The listing builds one solid part. Answer for the finished solid, in the listing's coordinates (mm). A direction names the side the tool comes from. Give positions to 0.01 mm unless a question says otherwise; leave off trailing zeros. Order: outer loops, then holes, each group sorted by start corner. A loop starts at its lowest first (then second) coordinate and runs counter-clockwise, first axis right, second up. Notation, with made-up numbers: (-16.75, -14.5) - (22.25, -14.5) arc R10 ccw to (22.25, 1.5) - close; hole circle Ø9 at (-2, 26.25). An arc over 180 degrees is marked (long way). Answer in a Markdown table with one row per item. Add a question column.
Autodesk Inventor part; units mm, degrees
ref_plane "YZ Plane" through (0, 0, 0) normal (1, 0, 0) x (0, 1, 0)
ref_plane "XZ Plane" through (0, 0, 0) normal (0, 1, 0) x (-1, 0, 0)
ref_plane "XY Plane" through (0, 0, 0) normal (0, 0, 1) x (1, 0, 0)
sketch "Sketch1" plane through (0, 0, 0) normal (0, 0, 1) x (1, 0, 0)
  line L0 (80, 30) -> (-80, 30)
  line L1 (-80, 30) -> (-80, -30)
  line L2 (-80, -30) -> (80, -30)
  line L3 (80, -30) -> (80, 30)
  line L4 (80, 30) -> (-80, -30) construction
  line L5 (-80, 30) -> (80, -30) construction
  line L6 (-20, -30) -> (-80, -30)
  line L7 (-80, -30) -> (-80, 30)
  line L8 (-80, 30) -> (-20, 30)
  line L9 (-20, 30) -> (-20, -30)
  line L10 (-20, -30) -> (-80, 30) construction
  line L11 (-80, -30) -> (-20, 30) construction
  line L12 (20, -30) -> (80, -30)
  line L13 (80, -30) -> (80, 30)
  line L14 (80, 30) -> (20, 30)
  line L15 (20, 30) -> (20, -30)
  line L16 (20, -30) -> (80, 30) construction
  line L17 (80, -30) -> (20, 30) construction
  line L18 (0, 30) -> (0, -30) construction
  point P0 (0, 0)
  point P1 (-50, 0)
  point P2 (50, 0)
  point P3 (20, 30)
  point P4 (20, -30)
  point P5 (-20, -30)
  point P6 (-20, 30)
  dimension "d0" = 160
  dimension "d1" = 60
  dimension "d2" = 40
extrude "Extrusion1" add sketch "Sketch1" along normal blind 10 contours L3 L2 L15 L0 | L9 L2 L1 L0
sketch "Sketch2" plane through (0, 0, 10) normal (0, 0, 1) x (1, 0, 0)
  line L0 (-80, -30) -> (-20, -30)
  line L1 (80, -24) -> (-80, -24)
  line L2 (-80, -24) -> (-80, -30)
  line L3 (-80, -30) -> (80, -30)
  line L4 (80, -30) -> (80, -24)
  line L5 (80, -24) -> (-80, -30) construction
  line L6 (-80, -24) -> (80, -30) construction
  line L7 (80, -30) -> (80, 30)
  point P0 (0, 0)
  point P1 (0, -27)
  dimension "d5" = 6
extrude "Extrusion2" add sketch "Sketch2" along normal blind 115
sketch "Sketch3" plane through (0, 0, 0) normal (0, 0, -1) x (-1, 0, 0)
  line L0 (53, 7.5) -> (43, 7.5)
  line L1 (43, 7.5) -> (43, -7.5)
  line L2 (43, -7.5) -> (53, -7.5)
  line L3 (53, -7.5) -> (53, 7.5)
  line L4 (53, 7.5) -> (43, -7.5) construction
  line L5 (43, 7.5) -> (53, -7.5) construction
  line L6 (-43, 7.5) -> (-53, 7.5)
  line L7 (-53, 7.5) -> (-53, -7.5)
  line L8 (-53, -7.5) -> (-43, -7.5)
  line L9 (-43, -7.5) -> (-43, 7.5)
  line L10 (-43, 7.5) -> (-53, -7.5) construction
  line L11 (-53, 7.5) -> (-43, -7.5) construction
  line L12 (80, -30) -> (-80, -30) construction
  line L13 (0, -30) -> (0, 0) construction
  point P0 (48, 0)
  point P1 (-48, 0)
  point P2 (48, 0)
  dimension "d8" = 10
  dimension "d9" = 15
  dimension "d10" = 48
extrude "Extrusion3" cut sketch "Sketch3" against normal through all
sketch "Sketch4" plane through (0, 0, 0) normal (0, 0, -1) x (-1, 0, 0)
  line L0 (-70, -20) -> (70, -20) construction
  line L1 (70, -20) -> (70, 20) construction
  line L2 (70, 20) -> (-70, 20) construction
  line L3 (-70, 20) -> (-70, -20) construction
  line L4 (-70, -20) -> (70, 20) construction
  line L5 (70, -20) -> (-70, 20) construction
  circle A0 centre (70, 20) radius 1.25
  circle A1 centre (-70, 20) radius 1.25
  circle A2 centre (-70, -20) radius 1.25
  circle A3 centre (70, -20) radius 1.25
  point P0 (0, 0)
  dimension "d13" = 140
  dimension "d14" = 40
  dimension "d16" = 2.5
extrude "Extrusion4" cut sketch "Sketch4" against normal through all
sketch "Sketch5" plane through (-20, -24, 10) normal (0, 1, 0) x (1, 0, 0)
  line L0 (59.5, -13) -> (-19.5, -13) construction
  line L1 (-19.5, -13) -> (-19.5, -113) construction
  line L2 (-19.5, -113) -> (59.5, -113) construction
  line L3 (59.5, -113) -> (59.5, -13) construction
  line L4 (59.5, -13) -> (-19.5, -113) construction
  line L5 (-19.5, -13) -> (59.5, -113) construction
  line L6 (100, -115) -> (-60, -115) construction
  line L7 (55.5, -17) -> (-2.5, -17) construction
  line L8 (-2.5, -17) -> (-2.5, -103) construction
  line L9 (-2.5, -103) -> (55.5, -103) construction
  line L10 (55.5, -103) -> (55.5, -17) construction
  line L11 (55.5, -17) -> (-2.5, -103) construction
  line L12 (-2.5, -17) -> (55.5, -103) construction
  circle A0 centre (-2.5, -17) radius 1.75
  circle A1 centre (55.5, -17) radius 1.75
  circle A2 centre (-2.5, -103) radius 1.75
  circle A3 centre (55.5, -103) radius 1.75
  line L13 (-60, -22) -> (-24, -22)
  line L14 (-24, -22) -> (-24, -98)
  line L15 (-24, -98) -> (-60, -98)
  line L16 (-60, -98) -> (-60, -22)
  line L17 (-60, -22) -> (-24, -98) construction
  line L18 (-24, -22) -> (-60, -98) construction
  line L19 (100, -22) -> (64, -22)
  line L20 (64, -22) -> (64, -98)
  line L21 (64, -98) -> (100, -98)
  line L22 (100, -98) -> (100, -22)
  line L23 (100, -22) -> (64, -98) construction
  line L24 (64, -22) -> (100, -98) construction
  line L25 (20, 10) -> (20, -115) construction
  line L26 (-60, 0) -> (-60, -115) construction
  circle A4 centre (-42, -16.5) radius 1.25
  circle A5 centre (-42, -103.5) radius 1.25
  circle A6 centre (82, -16.5) radius 1.25
  circle A7 centre (82, -103.5) radius 1.25
  line L27 (-60, 10) -> (-60, -115) construction
  line L28 (0, 0) -> (-60, 0)
  circle A8 centre (-2.5, -17) radius 3
  circle A9 centre (55.5, -17) radius 3
  circle A10 centre (-2.5, -103) radius 3
  circle A11 centre (55.5, -103) radius 3
  point P0 (20, -63)
  point P1 (20, -63)
  point P2 (26.5, -60)
  point P3 (20, -63)
  point P4 (26.5, -60)
  point P5 (-42, -60)
  point P6 (82, -60)
  point P7 (-42, -60)
  point P8 (82, -60)
  point P9 (-42, -60)
  point P10 (82, -60)
  dimension "d20" = 79
  dimension "d21" = 100
  dimension "d22" = 58
  dimension "d23" = 86
  dimension "d26" = 4
  dimension "d27" = 4
  dimension "d28" = 3.5
  dimension "d31" = 36
  dimension "d32" = 76
  dimension "d36" = 2.5
  dimension "d39" = 13
  dimension "d42" = 4.5
  dimension "d45" = 6
  dimension "d50" = 43.5
  dimension "d51" = 43.5
  dimension "d52" = 55
extrude "Extrusion5" cut sketch "Sketch5" against normal through all contours A0 | A1 | A2 | A3
extrude "Extrusion6" cut sketch "Sketch5" against normal through all contours L13 L14 L15 L16 | L22 L21 L20 L19
extrude "Extrusion7" cut sketch "Sketch5" against normal through all contours A4 | A5 | A6 | A7
extrude "Extrusion8" add sketch "Sketch5" along normal blind 4 contours A8 | A9 | A10 | A11
fillet "Fillet1" radius 1 4 edges at (-25.5, -24, 27) (32.5, -24, 27) (-25.5, -24, 113) (32.5, -24, 113)
properties part number "electrical_system_fix_board"
(1) Each of these flat-tipped pins is pushed along its axis until it touches: P1, Ø6.5, axis at x = 35.5, z = 27, coming from the +Y side; P2, Ø10, axis at x = 33.5, y = -14.5, coming from the +Z side; P3, Ø2, axis at x = -70, y = 20, coming from the +Z side; P4, Ø3, axis at x = 8.5, y = -26.5, coming from the -Z side. Where does it stop, or does it pass through?
(2) Find section B-B, the plane z = 41. Write down the section's boundary in (x, y), plus the area to 3 significant figures.
(3) Find section A-A, the plane y = 16. Write down the section's boundary in (x, z), plus the area to 3 significant figures.
(4) Straight lines are drawn through the part: line 1 (Y direction, x = -70, z = 2); line 2 (Z direction, x = 62, y = -27.95); line 3 (Z direction, x = -41, y = 10.5). For each, find the intervals that lie inside material, in ascending order.
(5) The mould has two halves that part along Y. Classify faces 6 (the face through (53, 0, 5)), 7 (the face through (-50, 30, 5)), 8 (the face through (-62, -27, 108)): +Y half, -Y half, draft (parallel to the pull), parting line (faces both ways), or undercut.
(6) For faces 1 (the face through (-25.5, -21.5, 27.1)), 2 (the face through (44, -27, 69)), 3 (the face through (37.5, -20, 27)), 4 (the face through (-48, -7.5, 5)), 5 (the face through (-62, -27, 32)), determine the directions among +Z, -Z, +X, -X, +Y, -Y from which every point of the face is accessible in a straight line to the end or side of a thin tool.
Answer key:
| question | item | result |
|---|---|---|
| 1 | P1 | y = -20 |
| 1 | P2 | z = 10 |
| 1 | P3 | through |
| 1 | P4 | z = 10 |
| 2 | outline | (-44, -30) - (44, -30) - (44, -24) - (-44, -24) - close |
| 2 | area | 528 mm² |
| 3 | outline | (-80, 0) - (-20, 0) - (-20, 10) - (-80, 10) - close; (20, 0) - (80, 0) - (80, 10) - (20, 10) - close |
| 3 | area | 1,200 mm² |
| 4 | line 1 | -30 to -21.25, -18.75 to 18.75, 21.25 to 30 |
| 4 | line 2 | 0 to 25.25, 27.75 to 32, 108 to 112.25, 114.75 to 125 |
| 4 | line 3 | 0 to 10 |
| 5 | face 6 | undercut |
| 5 | face 7 | +Y half |
| 5 | face 8 | draft |
| 6 | face 1 | +Y |
| 6 | face 2 | +X, +Y, -Y |
| 6 | face 3 | +Z, +X, -X, +Y |
| 6 | face 4 | +Z, -Z |
| 6 | face 5 | -X, +Y, -Y |
